```python
from build123d import *

# Parameters (mm, degrees)
PAD_DEPTH           = 10
LINEARPATTERN_COUNT = 4
LINEARPATTERN_PITCH = 10
SKETCH001_W         = 60
SKETCH001_H         = 3
PAD001_DEPTH        = 10
SKETCH002_R         = 2
POCKET_DEPTH        = 3


with BuildPart() as part:
    # Sketch → Pad (new body)
    with BuildSketch(Plane.XY):
        with BuildLine():
            Line((-5, 3), (5, 3))
            Line((5, 3), (5, 0))
            Line((5, 0), (2.702486, 0))
            ThreePointArc((3.207107, -5.839305), (4.153937, -2.816025), (2.702486, 0))
            Line((3.207107, -5.839305), (2.5, -5.132198))
            ThreePointArc((2.5, -5.132198), (0, 0), (-2.5, -5.132198))
            Line((-3.207107, -5.839305), (-2.5, -5.132198))
            ThreePointArc((-2.702486, 0), (-4.153937, -2.816025), (-3.207107, -5.839305))
            Line((-5, 0), (-2.702486, 0))
            Line((-5, 3), (-5, 0))
        make_face()
    pad = extrude(amount=PAD_DEPTH)

    # LinearPattern: Pad ×4
    with Locations(*[(i * LINEARPATTERN_PITCH, 0, 0) for i in range(1, LINEARPATTERN_COUNT)]):
        add(pad)

    # Sketch001 → Pad001 (join)
    with BuildSketch(Plane.XY):
        with Locations((15, 1.5)):
            Rectangle(SKETCH001_W, SKETCH001_H)
    extrude(amount=PAD001_DEPTH)

    # Sketch002 → Pocket (cut)
    with BuildSketch(Plane.XZ):
        with Locations((-10, 5)):
            Circle(SKETCH002_R)
        with Locations((40, 5)):
            Circle(SKETCH002_R)
    extrude(amount=-POCKET_DEPTH, mode=Mode.SUBTRACT)


solid = part.part
```
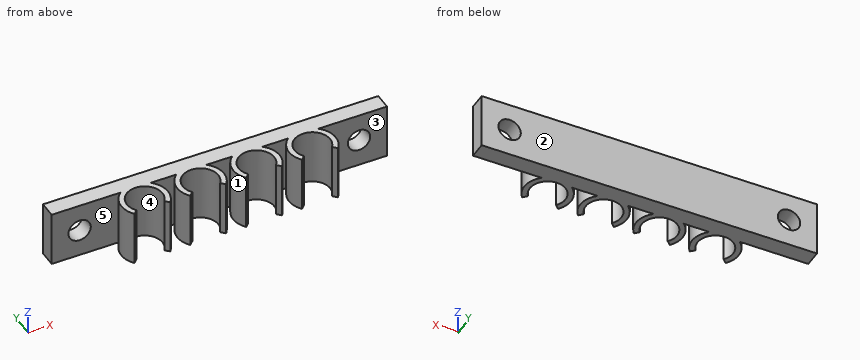
CAD build for the part. Positions are in the model's coordinates, mm. Face numbers are marked on the shaded views. A direction names the side the tool comes from. Round coordinates to 2 decimals unless told otherwise and drop trailing zeros. Write each loop counter-clockwise with the first axis right and the second up, starting at its lowest first coordinate (ties: lowest second). Pieces come first, ordered by that corner, then holes. Notation, with made-up numbers: (-15.75, -30.5) - (25.25, -30.5) arc R17 cw to (25.25, -10.5) - close; hole circle Ø6 at (44, 23). An arc over 180 degrees is marked (long way). Return JSON: item names as keys, results as strings. Group by question number.
Item 1: Band-saw the part on A-A on x = 40. List the corners of the cut face in (y, z).
Item 2: Probe probe 1 along X at (y, z) = (0.25, 3.25); probe 2 along Z at (x, y) = (40, 2.2); probe 3 along Y at (x, z) = (-8.5, 1). List the from-to ranges inside material, lowest first.
Item 3: 3-axis set-ups, long thin cutter, end or side, ignore diameter. For the marked faces 3, 4 and 5: which of +Z, -Z, +X, -X, +Y, -Y reach the whole face in a straight line?
Item 4: Band-saw the part on C-C on z = 2.5. List the corners of the cut face in (x, y) (3 decimals).
Item 5: Band-saw the part on B-B on y = -1.5. State how many separate pieces and enclosed holes the cut face has, plus the area to 3 significant figures.
Item 6: Flat gauge pins, fed straight in: pin 1 Ø1.4 at (x, z) = (6, 6.5) entering from -Y; pin 2 Ø3.5 at (x, z) = (25, 6) entering from -Y; pin 3 Ø4 at (y, z) = (-1.5, 5.5) entering from -X; pin 4 Ø3 at (x, z) = (37, 6) entering from -Y. Where does each tip first touch, or does it go through?
Item 7: Mould opens along X. For the marked faces 1 and 2 say: +X half, -X half, draft (parallel to the pull), parting line (faces both ways), or undercut.
Item 8: Band-saw the part on D-D on x = 0. List the corners of the cut face in (y, z).
Resolved:
{
 "1": {"outline": "(0, 0) - (3, 0) - (3, 3) - (0, 3) - close; (0, 7) - (3, 7) - (3, 10) - (0, 10) - close"},
 "2": {"probe 1": "x = -15 to -10.97, -9.03 to 39.03, 40.97 to 45", "probe 2": "z = 0 to 3, 7 to 10", "probe 3": "y = 0 to 3"},
 "3": {"face 3": "+Z, -Z, +X", "face 4": "+Z, -Z", "face 5": "+Z, -Z, -X"},
 "4": {"outline": "(-15, 0) - (-2.702, 0) arc R4.169 ccw to (-3.207, -5.839) - (-2.5, -5.132) arc R3.175 cw (long way) to (2.5, -5.132) - (3.207, -5.839) arc R4.169 ccw to (2.702, 0) - (7.298, 0) arc R4.169 ccw to (6.793, -5.839) - (7.5, -5.132) arc R3.175 cw (long way) to (12.5, -5.132) - (13.207, -5.839) arc R4.169 ccw to (12.702, 0) - (17.298, 0) arc R4.169 ccw to (16.793, -5.839) - (17.5, -5.132) arc R3.175 cw (long way) to (22.5, -5.132) - (23.207, -5.839) arc R4.169 ccw to (22.702, 0) - (27.298, 0) arc R4.169 ccw to (26.793, -5.839) - (27.5, -5.132) arc R3.175 cw (long way) to (32.5, -5.132) - (33.207, -5.839) arc R4.169 ccw to (32.702, 0) - (45, 0) - (45, 3) - (-15, 3) - close"},
 "5": {"separate pieces": "8", "enclosed holes": "0", "area": "89.7 mm²"},
 "6": {"pin 1": "stops at y = -5.72", "pin 2": "stops at y = -5.79", "pin 3": "stops at x = -15", "pin 4": "stops at y = 0"},
 "7": {"face 1": "undercut", "face 2": "draft"},
 "8": {"outline": "(0, 0) - (3, 0) - (3, 10) - (0, 10) - close"}
}
